```python
from build123d import *

# Parameters (mm, degrees)
SKETCH2_W               = 165
SKETCH2_H               = 117
BOSS_EXTRUDE1_DEPTH     = 4.5
SKETCH3_R               = 1.75
CUT_EXTRUDE1_DEPTH      = 5.5
MIRROR2_COPY_1_SKETCH_R = 1.75
MIRROR2_COPY_1_DEPTH    = 5.5
CUT_EXTRUDE2_REACH      = 6.5
SKETCH4_W               = 6
SKETCH4_H               = 16
CUT_EXTRUDE3_DEPTH      = 4.5


with BuildPart() as part:
    # Sketch2 → Boss-Extrude1 (new body)
    with BuildSketch(Plane.XY):
        Rectangle(SKETCH2_W, SKETCH2_H)
    extrude(amount=BOSS_EXTRUDE1_DEPTH)

    # Sketch3 → Cut-Extrude1 (cut, through all)
    with BuildSketch(Plane.XY.offset(4.5)):
        with Locations((-56.5, 44)):
            Circle(SKETCH3_R)
    cut_extrude1 = extrude(amount=-CUT_EXTRUDE1_DEPTH, mode=Mode.SUBTRACT)

    # Mirror1: Cut-Extrude1 across plane
    add(cut_extrude1.mirror(Plane(origin=(0, 0, 0), x_dir=(0, 0, 1), z_dir=(1, 0, 0))), mode=Mode.SUBTRACT)

    # Mirror2: Cut-Extrude1 across plane
    add(cut_extrude1.mirror(Plane.ZX), mode=Mode.SUBTRACT)

    # Mirror2 copy 1 sketch → Mirror2 copy 1 (cut, through all)
    with BuildSketch(Plane(origin=(0, 0, 4.5), x_dir=(-1, 0, 0), z_dir=(0, 0, 1))):
        with Locations((-56.5, 44)):
            Circle(MIRROR2_COPY_1_SKETCH_R)
    extrude(amount=-MIRROR2_COPY_1_DEPTH, mode=Mode.SUBTRACT)

    # Sketch4 → Cut-Extrude2 (cut, up to next)
    with BuildSketch(Plane.XY.offset(4.5), mode=Mode.PRIVATE) as cut_extrude2_sk1:
        with Locations((-67.5, 0)):
            Rectangle(SKETCH4_W, SKETCH4_H)
    cut_extrude2_tool1 = extrude(cut_extrude2_sk1.sketch, amount=-CUT_EXTRUDE2_REACH, mode=Mode.PRIVATE) & part.part
    add(cut_extrude2_tool1.solids().sort_by_distance((-67.5, 0, 4.5))[0], mode=Mode.SUBTRACT)

    # Sketch5 → Cut-Extrude3 (cut)
    with BuildSketch(Plane.XY.offset(4.5)):
        with BuildLine():
            ThreePointArc((-82.5, 49.340007913), (-81.621787101, 51.460201405), (-79.501593608, 52.338414304))
            Line((-79.501593608, 52.338414304), (-72.492625761, 52.338414304))
            ThreePointArc((-72.492625761, 52.338414304), (-69.498148124, 53.179301378), (-67.379159906, 55.456114132))
            ThreePointArc((-67.379159906, 55.456114132), (-66.828268927, 56.933959128), (-66.641125435, 58.5))
            Line((-66.641125435, 58.5), (-82.5, 58.5))
            Line((-82.5, 58.5), (-82.5, 49.340007913))
        make_face()
    cut_extrude3 = extrude(amount=-CUT_EXTRUDE3_DEPTH, mode=Mode.SUBTRACT)

    # Mirror3: Cut-Extrude3 across plane
    add(cut_extrude3.mirror(Plane.ZX), mode=Mode.SUBTRACT)


solid = part.part
```
Work out the finished part from the listing and answer in its coordinate system (mm). A direction names the side the tool comes from. Round coordinates to 2 decimals unless told otherwise and drop trailing zeros. Write each loop counter-clockwise with the first axis right and the second up, starting at its lowest first coordinate (ties: lowest second). Pieces come first, ordered by that corner, then holes.
1) Which of the six approach directions +Z, -Z, +X, -X, +Y, -Y give full straight-line access (tool end or side, diameter ignored) to faces 4 (the face through (-1, 1, 0)), 5 (the face through (-76, 52.338, 2)), 6 (the face through (-68, 8, 2))?
2) Determine the mould class of faces 1 (the face through (54.883, -43.33, 2.282)), 2 (the face through (-66.834, -56.912, 2.282)), 3 (the face through (-76, -52.338, 2)) for opening direction X: pulls with the +X half, pulls with the -X half, needs draft (parallel to the pull), parting line crosses it, or undercut.
3) A cutting plane is placed at A-A on y = -44. Determine the outline of the cut face in (x, z).
4) Flat-ended cylindrical pins translate along their axes: P1, Ø5.5, axis at x = 56.5, y = 44, coming from the -Z side; P2, Ø2, axis at x = -76.5, z = 1, coming from the -Y side. Find the tip coordinate at first contact, or state that the pin passes through.
5) A cutting plane is placed at C-C on x = -56.5. Determine the outline of the cut face in (y, z).
6) Consider probe 1 along Y at (x, z) = (56.5, 3.05); probe 2 along X at (y, z) = (-44, 2.6); probe 3 along X at (y, z) = (-43, 2.4). Determine where each line is inside the solid, lowest interval first.
7) A cutting plane is placed at B-B on z = 2.35. Determine the outline of the cut face in (x, y), and give its area (3 significant figures).
Entries:
1. face 4: -Z, +X, -X, +Y, -Y
1. face 5: +Z, -Z, -X, +Y
1. face 6: +Z, -Z
2. face 1: undercut
2. face 2: pulls with the -X half
2. face 3: needs draft
3. outline: (-82.5, 0) - (-58.25, 0) - (-58.25, 4.5) - (-82.5, 4.5) - close; (-54.75, 0) - (54.75, 0) - (54.75, 4.5) - (-54.75, 4.5) - close; (58.25, 0) - (82.5, 0) - (82.5, 4.5) - (58.25, 4.5) - close
4. P1: stops at z = 0
4. P2: stops at y = -52.34
5. outline: (-58.5, 0) - (-45.75, 0) - (-45.75, 4.5) - (-58.5, 4.5) - close; (-42.25, 0) - (42.25, 0) - (42.25, 4.5) - (-42.25, 4.5) - close; (45.75, 0) - (58.5, 0) - (58.5, 4.5) - (45.75, 4.5) - close
6. probe 1: y = -58.5 to -45.75, -42.25 to 42.25, 45.75 to 58.5
6. probe 2: x = -82.5 to -58.25, -54.75 to 54.75, 58.25 to 82.5
6. probe 3: x = -82.5 to -57.94, -55.06 to 55.06, 57.94 to 82.5
7. outline: (-82.5, -49.34) arc R3 ccw to (-79.5, -52.34) - (-72.49, -52.34) arc R5.75 cw to (-67.38, -55.46) arc R6.65 cw to (-66.64, -58.5) - (82.5, -58.5) - (82.5, 58.5) - (-66.64, 58.5) arc R6.65 cw to (-67.38, 55.46) arc R5.75 cw to (-72.49, 52.34) - (-79.5, 52.34) arc R3 ccw to (-82.5, 49.34) - close; hole (-70.5, -8) - (-64.5, -8) - (-64.5, 8) - (-70.5, 8) - close; hole circle Ø3.5 at (-56.5, -44); hole circle Ø3.5 at (-56.5, 44); hole circle Ø3.5 at (56.5, -44); hole circle Ø3.5 at (56.5, 44)
7. area: 19,000 mm2
